```python
from build123d import *

# Parameters (mm, degrees)
F0_W          = 6.35
F0_H          = 25.4
F3_W          = 6.35
F3_H          = 25.4
F3_R          = 3.301997
F4_DEPTH      = 6.35
F4_DEPTH_BACK = 6.35


with BuildPart() as f2:
    # F0 (on Front) → F2 (revolve)
    with BuildSketch(Plane.XZ):
        with Locations((-15.875, 12.7)):
            Rectangle(F0_W, F0_H)
    revolve(axis=Axis((0, 0, 24.002999), (0, 0, 1)))

    # F3 (on Front) → F4 (join, two sides)
    with BuildSketch(Plane.XZ) as f4_sk:
        with Locations((15.875, 12.7)):
            Rectangle(F3_W, F3_H)
        with BuildLine():
            ThreePointArc((19.05, 0), (31.75, 12.7), (19.05, 25.4))
            Line((19.05, 25.4), (19.05, 0))
        make_face()
        with Locations((25.4, 12.7)):
            Circle(F3_R, mode=Mode.SUBTRACT)
    extrude(amount=F4_DEPTH)
    extrude(f4_sk.sketch, amount=-F4_DEPTH_BACK)


solid = f2.part
```
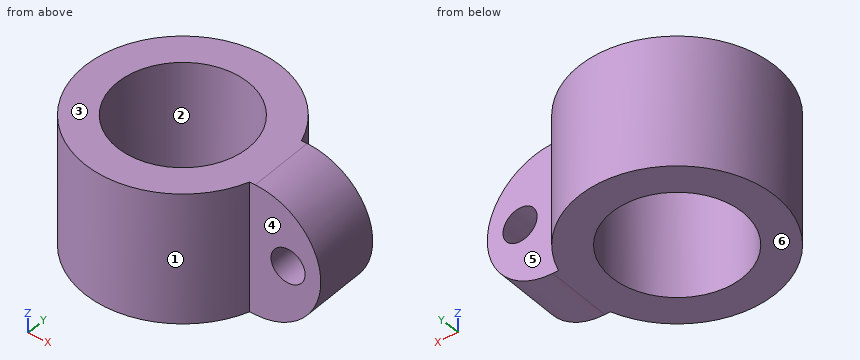
Part model, mm, in its own coordinate system. Face numbers are marked on the shaded views. A direction names the side the tool comes from. Round coordinates to 2 decimals unless told otherwise and drop trailing zeros. Write each loop counter-clockwise with the first axis right and the second up, starting at its lowest first coordinate (ties: lowest second). Pieces come first, ordered by that corner, then holes. Notation, with made-up numbers: M 61,73 L 101,73 A23 cw 101,107 Z; hole C 3.25,-34 d7. An arc over 180 degrees is marked long. One line per question, with ' | ' between items.
(1) Saw through at D-D on y = 7. Write the cut outline in (x, z), then the cut area to 3 significant figures.
Answer key:
outline: M -17.72,0 L -10.6,0 L -10.6,25.4 L -17.72,25.4 Z; M 10.6,0 L 17.72,0 L 17.72,25.4 L 10.6,25.4 Z | area: 362 mm^2
(2) Two-plate mould, pull along X, no slides. Class the marked faces 1, 2 and 3: released by +X, released by -X, zero draft, split by the parting line, or undercut.
Answer key:
face 1: split by the parting line | face 2: undercut | face 3: zero draft
(3) 3-axis set-ups, long thin cutter, end or side, ignore diameter. For the marked faces 4, 5 and 6: which of +Z, -Z, +X, -X, +Y, -Y reach the whole face in a straight line?
Answer key:
face 4: +Z, -Z, +X, -Y | face 5: +Z, -Z, +X, +Y | face 6: -Z, +X, -X, +Y, -Y
(4) Probe line 1 along Y through (x, z) = (0, 13); line 2 along X through (y, z) = (0, 10.5); line 3 along X through (y, z) = (0, 11.25). List the from-to ranges inside material, lowest first.
Answer key:
line 1: y = -19.05 to -12.7, 12.7 to 19.05 | line 2: x = -19.05 to -12.7, 12.7 to 22.94, 27.86 to 31.56 | line 3: x = -19.05 to -12.7, 12.7 to 22.43, 28.37 to 31.67
(5) Pin check, flat tips, straight feed: pin 1 (8 mm diameter, centred on y = -9.5, z = 10.5, fed in from +X); pin 2 (1.5 mm diameter, centred on x = -11.5, z = 22.5, fed in from +Y); pin 3 (6 mm diameter, centred on y = -5, z = 5, fed in from -X); pin 4 (7 mm diameter, centred on x = 24.5, z = 12, fed in from +Y). Stop position of each tip, or through.
Answer key:
pin 1: stops at x = 31.75 | pin 2: stops at y = 15.73 | pin 3: stops at x = -18.94 | pin 4: stops at y = 6.35
(6) Saw through at A-A on z = 12.7. Write the cut outline in (x, y).
Answer key:
outline: M 17.96,-6.35 L 22.1,-6.35 L 22.1,6.35 L 17.96,6.35 A19.05 ccw long Z; M 28.7,-6.35 L 31.75,-6.35 L 31.75,6.35 L 28.7,6.35 Z; hole C 0,0 d25.4
(7) Saw through at B-B on y = 0. Write the cut outline in (x, z).
Answer key:
outline: M -19.05,0 L -12.7,0 L -12.7,25.4 L -19.05,25.4 Z; M 12.7,0 L 19.05,0 A12.7 ccw 19.05,25.4 L 12.7,25.4 Z; hole C 25.4,12.7 d6.6
(8) Saw through at C-C on x = 0. Write the cut outline in (y, z).
Answer key:
outline: M -19.05,0 L -12.7,0 L -12.7,25.4 L -19.05,25.4 Z; M 12.7,0 L 19.05,0 L 19.05,25.4 L 12.7,25.4 Z
